Autodesk Inventor part; units mm, degrees
ref_plane "YZ Plane" through (0, 0, 0) normal (1, 0, 0) x (0, 1, 0)
ref_plane "XZ Plane" through (0, 0, 0) normal (0, 1, 0) x (-1, 0, 0)
ref_plane "XY Plane" through (0, 0, 0) normal (0, 0, 1) x (1, 0, 0)
sketch "Sketch1" plane through (0, 0, 0) normal (0, 0, 1) x (1, 0, 0)
  circle A0 centre (-23.2983, 91.6967) radius 2.75
  circle A1 centre (0, 115) radius 20
  circle A2 centre (23.9017, 91.6967) radius 2.75
  circle A3 centre (23.9017, 138.8967) radius 2.75
  circle A4 centre (-23.2983, 138.8967) radius 2.75
  line L0 (-23.2983, 91.6967) -> (-23.2983, 81.6967)
  line L1 (-23.2983, 81.6967) -> (-33.2983, 81.6967)
  line L2 (23.9017, 138.8967) -> (23.9017, 148.8967)
  line L3 (23.9017, 148.8967) -> (33.9017, 148.8967)
  line L4 (-25.2983, 81.6967) -> (25.9017, 81.6967)
  line L5 (33.9017, 89.6967) -> (33.9017, 148.8967)
  line L6 (33.9017, 148.8967) -> (-33.2983, 148.8967)
  line L7 (-33.2983, 148.8967) -> (-33.2983, 89.6967)
  line L8 (-33.2983, 89.6967) -> (-25.2983, 81.6967)
  line L9 (25.9017, 81.6967) -> (33.9017, 89.6967)
  point P0 (0, 0)
  point P1 (33.9017, 81.6967)
  dimension "d0" = 10
  dimension "d1" = 10
  dimension "d2" = 10
  dimension "d3" = 10
  dimension "d4" = 8
  dimension "d5" = 8
  dimension "d6" = 8
  dimension "d7" = 8
extrude "Extrusion1" add sketch "Sketch1" along normal blind 3
sketch "Sketch2" plane through (0, 0, 3) normal (0, 0, 1) x (1, 0, 0)
  line L0 (33.9017, 148.8967) -> (-33.2983, 148.8967)
  line L1 (33.9017, 89.6967) -> (33.9017, 148.8967)
  line L2 (-33.2983, 148.8967) -> (33.9017, 148.8967)
  line L3 (33.9017, 148.8967) -> (33.9017, 145.8967)
  line L4 (33.9017, 145.8967) -> (-33.2983, 145.8967)
  line L5 (-33.2983, 145.8967) -> (-33.2983, 148.8967)
  point P0 (0, 0)
  dimension "d10" = 3
extrude "Extrusion2" add sketch "Sketch2" along normal blind 65
chamfer "Chamfer1" distance 8 angle 45 1 edges at (33.9017, 147.3967, 68)
chamfer "Chamfer2" distance 8 angle 45 1 edges at (-33.2983, 147.3967, 68)
sketch "Sketch3" plane through (-33.2983, 89.6967, 0) normal (-1, 0, 0) x (0, 0, 1)
  line L0 (3, 56.2) -> (60, 56.2)
  line L1 (3, 56.2) -> (3, 31.2)
  line L2 (3, 56.2) -> (3, 0)
  line L3 (3, 56.2) -> (19, 56.2)
  line L4 (19, 56.2) -> (3, 31.2)
  point P0 (0, -89.6967)
  dimension "d19" = 25
  dimension "d20" = 16
extrude "Extrusion3" add sketch "Sketch3" against normal blind 3
sketch "Sketch4" plane through (33.9017, 89.6967, 0) normal (1, 0, 0) x (0, 0, -1)
  line L0 (-19, 56.2) -> (-3, 56.2)
  line L1 (-19, 56.2) -> (-3, 31.2)
  line L2 (-3, 56.2) -> (-3, 31.2)
  point P0 (0, -89.6967)
extrude "Extrusion4" add sketch "Sketch4" against normal blind 3
sketch "Sketch5" plane through (-33.2983, 148.8967, 0) normal (0, 1, 0) x (1, 0, 0)
  line L0 (67.2, 0) -> (67.2, -60)
  line L1 (67.2, -60) -> (57.2, -60)
  line L2 (54.7, -60) -> (54.7, -60)
  line L3 (52.2, -57.5) -> (52.2, -12.5)
  line L4 (54.7, -10) -> (54.7, -10)
  line L5 (57.2, -12.5) -> (57.2, -57.5)
  line L6 (0, -19) -> (0, -60)
  line L7 (0, -60) -> (10, -60)
  line L8 (12.5, -60) -> (12.5, -60)
  line L9 (15, -57.5) -> (15, -12.5)
  line L10 (12.5, -10) -> (12.5, -10)
  line L11 (10, -12.5) -> (10, -57.5)
  arc A0 (12.5, -10) -> (10, -12.5) centre (12.5, -12.5) ccw
  arc A1 (15, -12.5) -> (12.5, -10) centre (12.5, -12.5) ccw
  arc A2 (12.5, -60) -> (15, -57.5) centre (12.5, -57.5) ccw
  arc A3 (10, -57.5) -> (12.5, -60) centre (12.5, -57.5) ccw
  arc A4 (52.2, -57.5) -> (54.7, -60) centre (54.7, -57.5) ccw
  arc A5 (54.7, -60) -> (57.2, -57.5) centre (54.7, -57.5) ccw
  arc A6 (57.2, -12.5) -> (54.7, -10) centre (54.7, -12.5) ccw
  arc A7 (54.7, -10) -> (52.2, -12.5) centre (54.7, -12.5) ccw
  point P0 (33.2983, 0)
  point P1 (52.2, -10)
  point P2 (52.2, -60)
  point P3 (57.2, -10)
  point P4 (15, -10)
  point P5 (10, -10)
  dimension "d25" = 10
  dimension "d26" = 5
  dimension "d27" = 50
  dimension "d28" = 10
  dimension "d29" = 5
  dimension "d30" = 2.5
extrude "Extrusion5" cut sketch "Sketch5" against normal through all
sketch "Sketch7" plane through (0, 0, 3) normal (0, 0, 1) x (1, 0, 0)
  line L0 (30.9017, 120.8967) -> (30.9017, 145.8967)
  line L1 (30.9017, 145.8967) -> (-30.2983, 145.8967)
  line L2 (-30.2983, 145.8967) -> (-30.2983, 120.8967)
  line L3 (-30.2983, 120.8967) -> (-33.2983, 120.8967)
  line L4 (-33.2983, 120.8967) -> (-33.2983, 89.6967)
  line L5 (-33.2983, 89.6967) -> (-25.2983, 81.6967)
  line L6 (-25.2983, 81.6967) -> (25.9017, 81.6967)
  line L7 (25.9017, 81.6967) -> (33.9017, 89.6967)
  line L8 (33.9017, 89.6967) -> (33.9017, 120.8967)
  line L9 (33.9017, 120.8967) -> (30.9017, 120.8967)
  circle A0 centre (0, 115) radius 20
  circle A1 centre (-23.2983, 138.8967) radius 2.75
  circle A2 centre (23.9017, 91.6967) radius 2.75
  circle A3 centre (23.9017, 138.8967) radius 2.75
  circle A4 centre (-23.2983, 91.6967) radius 2.75
  point P0 (0, 0)
equation "\"d5\" = d4"
properties part number "afirma_motor"
The model under review builds one solid part; all positions refer to its coordinate system, in mm. A direction names the side the tool comes from. Give positions to 0.01 mm unless a question says otherwise; leave off trailing zeros. Write each loop counter-clockwise with the first axis right and the second up, starting at its lowest first coordinate (ties: lowest second). Pieces come first, ordered by that corner, then holes. Notation, with made-up numbers: M 76.5,70 L 129.5,70 A27 cw 129.5,87 Z; hole C -31.75,50 d6. An arc over 180 degrees is marked long. One line per question, with ' | ' between items. Start each with the question number.
Item 1: We need section A-A on x = 0. Write out the cut boundary in (y, z).
Item 2: Draft analysis for pull direction X (two halves, no side actions). For faces 4 (the flat face through (15, 131, 0)), 5 (the cylindrical face through (-20.85, 147.42, 60)), 6 (the flat face through (-29.4, 147.4, 63.9)), 7 (the cylindrical face through (-20.7, 147.4, 10)), state which applies: released by +X, released by -X, zero draft, split by the parting line, or undercut.
Item 3: We need section D-D on y = 127.5. Write out the cut boundary in (x, z), plus the area to 3 significant figures.
Item 4: For faces 1 (the flat face through (-33.298, 137, 12)), 2 (the flat face through (-23.298, 147, 35)), 3 (the flat face through (-30.298, 136, 9)), list the 3-axis set-ups (+Z, -Z, +X, -X, +Y, -Y) from which the entire face can be reached by the end or side of a thin tool; tool diameter is ignored.
Item 5: For pin 1 (12 mm diameter, centred on x = -3.5, y = 104.5, fed in from -Z); pin 2 (7 mm diameter, centred on x = 23.9, y = 91.7, fed in from +Z); pin 3 (10 mm diameter, centred on x = 5, z = 49.5, fed in from -Y); pin 4 (6 mm diameter, centred on x = 19, z = 12, fed in from +Y), all flat-tipped, find the tip position at first contact; note any pin that passes through.
Item 6: We need section B-B on z = 38. Write out the cut boundary in (x, y).
Item 7: We need section C-C on y = 115. Write out the cut boundary in (x, z), plus the area to 3 significant figures.
Item 8: Wall thickness on line 1 (X direction, y = 146, z = 54); line 2 (X direction, y = 143.5, z = 5.5); line 3 (Y direction, x = -9.5, z = 36.5): over which ranges is each line inside the solid? List them lowest first. Write a range as from..to.
Results found:
1) outline: M 81.7,0 L 95,0 L 95,3 L 81.7,3 Z; M 135,0 L 148.9,0 L 148.9,68 L 145.9,68 L 145.9,3 L 135,3 Z
2) face 4: zero draft | face 5: undercut | face 6: released by -X | face 7: undercut
3) outline: M -33.3,0 L -15.61,0 L -15.61,3 L -30.3,3 L -30.3,7.23 L -33.3,7.23 Z; M 15.61,0 L 33.9,0 L 33.9,7.23 L 30.9,7.23 L 30.9,3 L 15.61,3 Z | area: 133 mm2
4) face 1: +Z, -Z, -X, +Y, -Y | face 2: +Y, -Y | face 3: +Z, -Y
5) pin 1: passes through | pin 2: stops at z = 3 | pin 3: stops at y = 145.9 | pin 4: stops at y = 148.9
6) outline: M -33.3,145.9 L -23.3,145.9 L -23.3,148.9 L -33.3,148.9 Z; M -18.3,145.9 L 18.9,145.9 L 18.9,148.9 L -18.3,148.9 Z; M 23.9,145.9 L 33.9,145.9 L 33.9,148.9 L 23.9,148.9 Z
7) outline: M -33.3,0 L -20,0 L -20,3 L -33.3,3 Z; M 20,0 L 33.9,0 L 33.9,3 L 20,3 Z | area: 81.6 mm2
8) line 1: x = -33.3..-23.3, -18.3..18.9, 23.9..33.9 | line 2: x = -33.3..-30.3, 30.9..33.9 | line 3: y = 145.9..148.9
